```python
from build123d import *

# Parameters (mm, degrees)
F0_W     = 7.1
F0_H     = 18
F1_DEPTH = 1.8
F0_W_2   = 2
F2_DEPTH = 8


# Not quite as in the source:
# - a feature names something its author has since deleted; it is built from what else it names


with BuildPart() as f1:
    # F0 (on Top) → F1 (new body)
    with BuildSketch(Plane.XY):
        Polygon((5.55, -9), (3.55, -9), (-3.55, -9), (-5.55, -9), (-5.55, -19), (5.55, -19), align=None)
        Rectangle(F0_W, F0_H)
        Polygon((-5.55, -19), (-5.55, -9), (-5.55, 9), (-11.55, 9), (-11.55, -19), align=None)
    extrude(amount=F1_DEPTH)

    # F0 (on Top) → F2 (join)
    with BuildSketch(Plane.XY):
        with Locations((-4.55, 0)):
            Rectangle(F0_W_2, F0_H)
        with Locations((4.55, 0)):
            Rectangle(F0_W_2, F0_H)
    extrude(amount=F2_DEPTH)


solid = f1.part
```
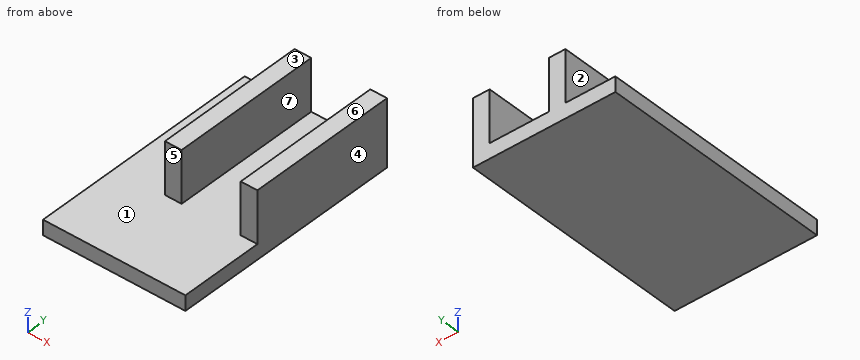
Check sheet for the modelled part. Datum: model origin and axes. Units: mm. Face numbers are marked on the shaded views. A direction names the side the tool comes from. Give positions to 0.01 mm unless a question says otherwise; leave off trailing zeros. Order: outer loops, then holes, each group sorted by start corner. A loop starts at its lowest first (then second) coordinate and runs counter-clockwise, first axis right, second up. Notation, with made-up numbers: M 31,-23 L 80,-23 A20 ccw 80,-6 Z; hole C 81.25,-37.5 d10. An arc over 180 degrees is marked long. Answer in a Markdown table with one row per item. Add a question column.
Q1. Sectioned sample at C-C, the plane x = 4.25. Record the boundary of the cut face in (y, z), and give its area (3 significant figures).
Q2. Release check for a two-part mould opening along X. For the marked faces 1, 2, 3 and 4 record: released by +X, released by -X, zero draft, split by the parting line, or undercut.
Q3. Access from +Z, -Z, +X, -X, +Y, -Y to the whole of each face (thin tool, end or side, straight path). Record for the marked faces 5, 6 and 7.
Q4. Sectioned sample at A-A, the plane z = 6.75. Record the boundary of the cut face in (x, y), and give its area (3 significant figures).
Q5. Sectioned sample at B-B, the plane y = 7. Record the boundary of the cut face in (x, z).
Q6. Gauge pin test, flat ends, axial feed: pin 1 Ø1 at (x, y) = (-3, -8) entering from +Z; pin 2 Ø2 at (x, z) = (3, 5) entering from -Y; pin 3 Ø1.9 at (y, z) = (3, 6) entering from -X. Record the tip position at first contact, or that the pin passes through.
Q7. Thickness scan on L1, parallel to X at y = -8.5, z = 2; L2, parallel to Z at x = 2.25, y = -7.75; L3, parallel to Y at x = -4.5, z = 3.5. Record the ranges inside material, lowest first.
Q8. Sectioned sample at D-D, the plane y = -11.5. Record the boundary of the cut face in (x, z), and give its area (3 significant figures).
Verdict:
| question | item | result |
|---|---|---|
| 1 | outline | M -19,0 L 9,0 L 9,8 L -9,8 L -9,1.8 L -19,1.8 Z |
| 1 | area | 162 mm² |
| 2 | face 1 | undercut |
| 2 | face 2 | released by -X |
| 2 | face 3 | zero draft |
| 2 | face 4 | released by +X |
| 3 | face 5 | +Z, +X, -X, -Y |
| 3 | face 6 | +Z, +X, -X, +Y, -Y |
| 3 | face 7 | +Z, +Y, -Y |
| 4 | outline | M -5.55,-9 L -3.55,-9 L -3.55,9 L -5.55,9 Z; M 3.55,-9 L 5.55,-9 L 5.55,9 L 3.55,9 Z |
| 4 | area | 72.0 mm² |
| 5 | outline | M -11.55,0 L 5.55,0 L 5.55,8 L 3.55,8 L 3.55,1.8 L -3.55,1.8 L -3.55,8 L -5.55,8 L -5.55,1.8 L -11.55,1.8 Z |
| 6 | pin 1 | z = 1.8 |
| 6 | pin 2 | y = -9 |
| 6 | pin 3 | x = -5.55 |
| 7 | L1 | -5.55 to -3.55, 3.55 to 5.55 |
| 7 | L2 | 0 to 1.8 |
| 7 | L3 | -9 to 9 |
| 8 | outline | M -11.55,0 L 5.55,0 L 5.55,1.8 L -11.55,1.8 Z |
| 8 | area | 30.8 mm² |
